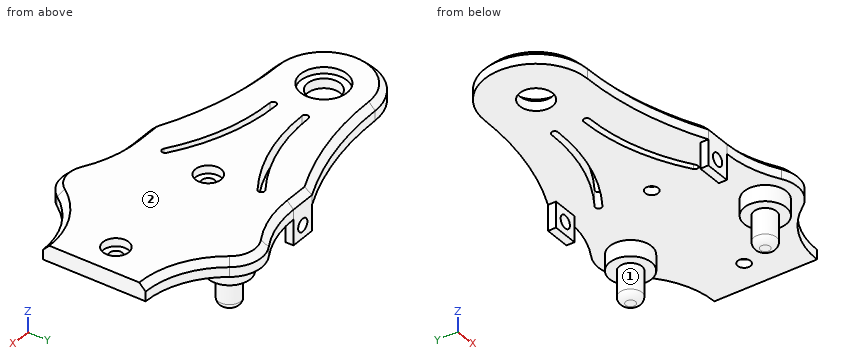
Autodesk Inventor part; units mm, degrees
ref_plane "YZ Plane" through (0, 0, 0) normal (1, 0, 0) x (0, 1, 0)
ref_plane "XZ Plane" through (0, 0, 0) normal (0, 1, 0) x (-1, 0, 0)
ref_plane "XY Plane" through (0, 0, 0) normal (0, 0, 1) x (1, 0, 0)
sketch "Sketch1" plane through (0, 0, 0) normal (0, 0, 1) x (1, 0, 0)
  circle A0 centre (0, 0) radius 5.08
  arc A1 (0, 16) -> (0, -16) centre (0, 0) ccw
  line L0 (0, 16) -> (99.4033, 16)
  line L1 (99.4033, 16) -> (99.4033, -16)
  line L2 (99.4033, -16) -> (0, -16)
  line L3 (0, -16) -> (0, 16) construction
  line L4 (39.8634, 25) -> (99.4033, 25)
  line L5 (99.4033, 25) -> (99.4033, -25)
  line L6 (99.4033, -25) -> (39.8634, -25)
  line L7 (39.8634, -25) -> (39.8634, 25)
  arc A2 (39.8634, -25) -> (0, -16) centre (0, -108.7828) ccw
  arc A3 (0, 16) -> (39.8634, 25) centre (0, 108.7828) ccw
  circle A4 centre (50.0625, 0) radius 2
  circle A5 centre (90.0625, 0) radius 2
  line L8 (-16, 0) -> (99.4033, 0) construction
  point P0 (39.8634, 0)
  dimension "d1" = 10.16
  dimension "d3" = 50
  dimension "d4" = 59.5399
  dimension "d12" = 4
  dimension "d13" = 40
  dimension "d14" = 50.0625
  dimension "d15" = 9.3408
  dimension "d44" = 16
extrude "Extrusion1" add sketch "Sketch1" along normal blind 5
ref_plane "Work Plane1" through (39.8634, 0, 0) normal (0, -1, 0) x (1, 0, 0)
sketch "Sketch4" plane through (0, 0, 5) normal (0, 0, 1) x (1, 0, 0)
  arc A0 (15, 6) -> (47.3064, 15.8305) centre (15, 64.0002) ccw
  arc A1 (15, 4) -> (48.4204, 14.1695) centre (15, 64.0002) ccw
  circle A2 centre (47.8634, 15) radius 1
  circle A3 centre (15, 5) radius 1
  arc A4 (0, 16) -> (39.8634, 25) centre (0, 108.7828) ccw
  line L0 (99.4033, 25) -> (39.8634, 25)
  line L1 (122.484, 0) -> (-39.0807, 0)
  line L2 (15, 4) -> (47.8634, 4) construction
  point P0 (0, 0)
  dimension "d16" = 2
  dimension "d17" = 10
  dimension "d18" = 8
  dimension "d19" = 15
  dimension "d20" = 5
extrude "Extrusion3" cut sketch "Sketch4" against normal through all
mirror "Mirror1" about plane through (39.8634, 0, 0) normal (0, -1, 0) of "Extrusion3"
sketch "Sketch5" plane through (0, 0, 0) normal (0, 0, -1) x (-1, 0, 0)
  arc A0 (-15, -4) -> (-48.4204, -14.1695) centre (-15, -64.0002) ccw
  arc A1 (-15, -6) -> (-15, -4) centre (-15, -5) ccw
  arc A2 (-15, -6) -> (-47.3064, -15.8305) centre (-15, -64.0002) ccw
  arc A3 (-48.4204, -14.1695) -> (-47.3064, -15.8305) centre (-47.8634, -15) ccw
  arc A4 (-47.3064, 15.8305) -> (-15, 6) centre (-15, 64.0002) ccw
  arc A5 (-15, 4) -> (-15, 6) centre (-15, 5) ccw
  arc A6 (-48.4204, 14.1695) -> (-15, 4) centre (-15, 64.0002) ccw
  arc A7 (-47.3064, 15.8305) -> (-48.4204, 14.1695) centre (-47.8634, 15) ccw
  arc A8 (0, -16) -> (0, 16) centre (0, 0) ccw
  arc A9 (-39.8634, 25) -> (0, 16) centre (0, 108.7828) ccw
  line L0 (-99.4033, 25) -> (-39.8634, 25)
  line L1 (-99.4033, -25) -> (-99.4033, 25)
  line L2 (-39.8634, -25) -> (-99.4033, -25)
  arc A10 (0, -16) -> (-39.8634, -25) centre (0, -108.7828) ccw
  circle A11 centre (-50.0625, 0) radius 2
  circle A12 centre (-90.0625, 0) radius 2
  circle A13 centre (0, 0) radius 5.08
  line L3 (-39.8634, 25) -> (-47.8634, 25)
  line L4 (-47.8634, 25) -> (-47.8634, 22.5)
  line L5 (-47.8634, 22.5) -> (-39.8634, 22.5)
  line L6 (-39.8634, 22.5) -> (-39.8634, 25)
  dimension "d23" = 8
  dimension "d24" = 2.5
extrude "Extrusion4" add sketch "Sketch5" along normal blind 8 contours L6 L5 L4 L0
sketch "Sketch6" plane through (39.8634, 25, 5) normal (0, 1, 0) x (1, 0, 0)
  line L0 (59.5399, 5) -> (8, 5)
  line L1 (8, 5) -> (8, 13)
  line L2 (0, 13) -> (8, 13)
  line L3 (0, 5) -> (0, 13)
  line L4 (0, 5) -> (0, 0)
  line L5 (59.5399, 0) -> (0, 0)
  line L6 (59.5399, 5) -> (59.5399, 0)
  circle A0 centre (4, 9) radius 2
  line L7 (4, 13) -> (4, 9) construction
  point P0 (-39.8634, 5)
  dimension "d27" = 4
  dimension "d28" = 4
extrude "Extrusion5" cut sketch "Sketch6" against normal up to next contours A0
mirror "Mirror2" about plane through (39.8634, 0, 0) normal (0, -1, 0) of "Extrusion4", "Extrusion5"
sketch "Sketch7" plane through (0, 0, 0) normal (0, 0, -1) x (-1, 0, 0)
  circle A0 centre (0, 0) radius 5.08
  circle A1 centre (-90.0625, 0) radius 2
  circle A2 centre (-50.0625, 0) radius 2
  arc A3 (-47.3064, 15.8305) -> (-15, 6) centre (-15, 64.0002) ccw
  arc A4 (-15, 4) -> (-15, 6) centre (-15, 5) ccw
  arc A5 (-48.4204, 14.1695) -> (-15, 4) centre (-15, 64.0002) ccw
  arc A6 (-47.3064, 15.8305) -> (-48.4204, 14.1695) centre (-47.8634, 15) ccw
  arc A7 (-15, -4) -> (-48.4204, -14.1695) centre (-15, -64.0002) ccw
  arc A8 (-15, -6) -> (-15, -4) centre (-15, -5) ccw
  arc A9 (-15, -6) -> (-47.3064, -15.8305) centre (-15, -64.0002) ccw
  arc A10 (-48.4204, -14.1695) -> (-47.3064, -15.8305) centre (-47.8634, -15) ccw
  line L0 (-47.8634, -25) -> (-47.8634, -22.5)
  line L1 (-47.8634, -22.5) -> (-39.8634, -22.5)
  line L2 (-39.8634, -22.5) -> (-39.8634, -25)
  arc A11 (0, -16) -> (-39.8634, -25) centre (0, -108.7828) ccw
  arc A12 (0, -16) -> (0, 16) centre (0, 0) ccw
  arc A13 (-39.8634, 25) -> (0, 16) centre (0, 108.7828) ccw
  line L3 (-39.8634, 25) -> (-39.8634, 22.5)
  line L4 (-39.8634, 22.5) -> (-47.8634, 22.5)
  line L5 (-47.8634, 22.5) -> (-47.8634, 25)
  line L6 (-99.4033, 25) -> (-47.8634, 25)
  line L7 (-99.4033, -25) -> (-99.4033, 25)
  line L8 (-47.8634, -25) -> (-99.4033, -25)
  circle A14 centre (-70.0625, 21) radius 10
  arc A15 (-65.0249, 29.6384) -> (-47.8634, 25) centre (-47.8634, 59.0667) ccw
  line L9 (-99.4033, 25) -> (-47.8634, 25)
  line L10 (39.0807, 0) -> (-122.484, 0)
  line L11 (-70.0625, -25) -> (-70.0625, 21) construction
  line L12 (-90.0625, 0) -> (-50.0625, 0) construction
  line L13 (0, 16) -> (-99.4033, 16) construction
  arc A16 (-99.4033, 16) -> (-78.1686, 26.8559) centre (-99.4033, 42.1961) ccw
  point P0 (-92.2616, 25)
  point P1 (-75.1001, 29.6384)
  point P2 (-70.0625, 0)
  point P3 (-60.8973, 25)
  point P4 (-79.2277, 25)
  point P5 (-79.6415, 25)
  dimension "d31" = 20
  dimension "d32" = 21
extrude "Extrusion6" add sketch "Sketch7" against normal up to surface (5 mm away) contours L6 A14 A15 | L6 A14 | A16 A14 L6 picked at (-67.4658, 26.7505)
sketch "Sketch8" plane through (0, 0, 0) normal (0, 0, -1) x (-1, 0, 0)
  circle A0 centre (0, 0) radius 5.08
  circle A1 centre (-90.0625, 0) radius 2
  circle A2 centre (-50.0625, 0) radius 2
  arc A3 (-47.3064, 15.8305) -> (-15, 6) centre (-15, 64.0002) ccw
  arc A4 (-15, 4) -> (-15, 6) centre (-15, 5) ccw
  arc A5 (-48.4204, 14.1695) -> (-15, 4) centre (-15, 64.0002) ccw
  arc A6 (-47.3064, 15.8305) -> (-48.4204, 14.1695) centre (-47.8634, 15) ccw
  arc A7 (-15, -4) -> (-48.4204, -14.1695) centre (-15, -64.0002) ccw
  arc A8 (-15, -6) -> (-15, -4) centre (-15, -5) ccw
  arc A9 (-15, -6) -> (-47.3064, -15.8305) centre (-15, -64.0002) ccw
  arc A10 (-48.4204, -14.1695) -> (-47.3064, -15.8305) centre (-47.8634, -15) ccw
  line L0 (-47.8634, -25) -> (-47.8634, -22.5)
  line L1 (-47.8634, -22.5) -> (-39.8634, -22.5)
  line L2 (-39.8634, -22.5) -> (-39.8634, -25)
  arc A11 (0, -16) -> (-39.8634, -25) centre (0, -108.7828) ccw
  arc A12 (0, -16) -> (0, 16) centre (0, 0) ccw
  arc A13 (-39.8634, 25) -> (0, 16) centre (0, 108.7828) ccw
  line L3 (-39.8634, 25) -> (-39.8634, 22.5)
  line L4 (-39.8634, 22.5) -> (-47.8634, 22.5)
  line L5 (-47.8634, 22.5) -> (-47.8634, 25)
  arc A14 (-65.0249, 29.6384) -> (-47.8634, 25) centre (-47.8634, 59.0667) ccw
  arc A15 (-65.0249, 29.6384) -> (-78.1686, 26.8559) centre (-70.0625, 21) ccw
  line L6 (-99.4033, 25) -> (-79.6415, 25)
  line L7 (-99.4033, -25) -> (-99.4033, 25)
  line L8 (-47.8634, -25) -> (-99.4033, -25)
  circle A16 centre (-70.0625, 21) radius 6.5
  arc A17 (-79.6415, 25) -> (-78.1686, 26.8559) centre (-99.4033, 42.1961) ccw
  dimension "d35" = 13
extrude "Extrusion7" add sketch "Sketch8" along normal blind 5 contours A16
sketch "Sketch9" plane through (70.0625, 21, -5) normal (0, 0, -1) x (-1, 0, 0)
  circle A0 centre (0, 0) radius 3.5
  circle A1 centre (0, 0) radius 6.5
  point P0 (70.0625, -21)
  dimension "d38" = 7
extrude "Extrusion8" add sketch "Sketch9" along normal blind 10 contours A0
fillet "Fillet1" radius 2 1 edges at (73.5625, 21, -15)
extrude "Extrusion9" cut sketch "Sketch7" against normal through all contours L7 L6 A16
mirror "Mirror3" about plane through (39.8634, 0, 0) normal (0, -1, 0) of "Extrusion6", "Extrusion7", "Extrusion8", "Fillet1", "Extrusion9"
sketch "Sketch10" plane through (0, 0, 5) normal (0, 0, 1) x (1, 0, 0)
  arc A0 (48.4204, -14.1695) -> (15, -4) centre (15, -64.0002) ccw
  arc A1 (47.3064, -15.8305) -> (48.4204, -14.1695) centre (47.8634, -15) ccw
  arc A2 (47.3064, -15.8305) -> (15, -6) centre (15, -64.0002) ccw
  arc A3 (15, -4) -> (15, -6) centre (15, -5) ccw
  arc A4 (15, 6) -> (47.3064, 15.8305) centre (15, 64.0002) ccw
  arc A5 (48.4204, 14.1695) -> (47.3064, 15.8305) centre (47.8634, 15) ccw
  arc A6 (15, 4) -> (48.4204, 14.1695) centre (15, 64.0002) ccw
  arc A7 (15, 6) -> (15, 4) centre (15, 5) ccw
  arc A8 (99.4033, -16) -> (78.1686, -26.8559) centre (99.4033, -42.1961) ccw
  line L0 (99.4033, -16) -> (99.4033, 16)
  arc A9 (78.1686, 26.8559) -> (99.4033, 16) centre (99.4033, 42.1961) ccw
  line L1 (47.8634, 25) -> (39.8634, 25)
  arc A10 (78.1686, 26.8559) -> (65.0249, 29.6384) centre (70.0625, 21) ccw
  arc A11 (47.8634, 25) -> (65.0249, 29.6384) centre (47.8634, 59.0667) ccw
  arc A12 (0, 16) -> (39.8634, 25) centre (0, 108.7828) ccw
  arc A13 (0, 16) -> (0, -16) centre (0, 0) ccw
  arc A14 (39.8634, -25) -> (0, -16) centre (0, -108.7828) ccw
  line L2 (39.8634, -25) -> (47.8634, -25)
  arc A15 (65.0249, -29.6384) -> (47.8634, -25) centre (47.8634, -59.0667) ccw
  arc A16 (65.0249, -29.6384) -> (78.1686, -26.8559) centre (70.0625, -21) ccw
  circle A17 centre (50.0625, 0) radius 2
  circle A18 centre (90.0625, 0) radius 2
  circle A19 centre (0, 0) radius 5.08
  circle A20 centre (50.0625, 0) radius 4
  circle A21 centre (90.0625, 0) radius 4
  dimension "d45" = 8
extrude "Extrusion10" cut sketch "Sketch10" against normal blind 2.5 contours A20 | A21
sketch "Sketch11" plane through (0, 0, 5) normal (0, 0, 1) x (1, 0, 0)
  circle A0 centre (0, 0) radius 7.235
  dimension "d48" = 14.47
extrude "Extrusion11" cut sketch "Sketch11" against normal blind 2
chamfer "Chamfer1" distance 2 angle 45 5 edges at (20.4334, 18.278, 5) (-16, 0, 5) (20.4334, -18.278, 5) (43.8634, 25, 5) (43.8634, -25, 5)
properties part number "Bearing_Arm_2"
Design review of the part built by this model. Coordinates are the model's own, in mm. Face numbers are marked on the shaded views. Give positions to 0.01 mm unless a question says otherwise; leave off trailing zeros. Order: outer loops, then holes, each group sorted by start corner. A loop starts at its lowest first (then second) coordinate and runs counter-clockwise, first axis right, second up. Notation, with made-up numbers: (66.5, 81) - (81.5, 81) arc R22 ccw to (81.5, 103) - close; hole circle Ø7 at (-16.5, -18). An arc over 180 degrees is marked (long way). Use a Markdown table: item, result. Add a question column.
(1) Clearance check with flat-ended pins moving along their axes: P1, Ø5, axis at y = -20.5, z = 1.5, coming from the +X side; P2, Ø5, axis at x = 43.86, z = -4, coming from the +Y side; P3, Ø3, axis at x = 42.5, y = -23.5, coming from the -Z side. State where each tip first meets the part, or that it passes through.
(2) Add section B-B on x = 30.5. Give the number of separate pieces and of enclosed holes in the cut face, then the cut area to 3 significant figures.
(3) Add section A-A on z = -10.5. Give the boundary of the cut face in (x, y).
(4) Wall thickness on probe 1 along Y at (x, z) = (0, 0.7); probe 2 along Z at (x, y) = (30.5, -15); probe 3 along X at (y, z) = (23.4, -4): over which ranges is each line inside the solid? List them lowest first. Write a range as [from, to].
(5) Mouldability with a two-part tool opening along Y and no side actions: class the marked faces 1 and 2 as +Y half, -Y half, draft (parallel to the pull), parting line (faces both ways), or undercut.
Report:
| question | item | result |
|---|---|---|
| 1 | P1 | stops at x = 89.36 |
| 1 | P2 | stops at y = 25 |
| 1 | P3 | stops at z = -8 |
| 2 | separate pieces | 3 |
| 2 | enclosed holes | 0 |
| 2 | area | 187 mm² |
| 3 | outline | circle Ø7 at (70.06, -21); circle Ø7 at (70.06, 21) |
| 4 | probe 1 | y = [-16, -5.08], [5.08, 16] |
| 4 | probe 2 | z = [0, 5] |
| 4 | probe 3 | x = [39.86, 41.86], [45.86, 47.86], [64.02, 76.1] |
| 5 | face 1 | undercut |
| 5 | face 2 | draft |
